The listing builds one solid part. Answer for the finished solid, in the listing's coordinates (mm). A direction names the side the tool comes from. Round coordinates to 2 decimals unless told otherwise and drop trailing zeros. Order: outer loops, then holes, each group sorted by start corner. A loop starts at its lowest first (then second) coordinate and runs counter-clockwise, first axis right, second up. Notation, with made-up numbers: (25, -9) - (62, -9) arc R27 ccw to (62, 13) - close; hole circle Ø7 at (64, 69). An arc over 180 degrees is marked (long way). Write item = value, one per line.
from build123d import *

# Parameters (mm, degrees)
SKETCH1_R           = 8
SKETCH1_R_2         = 3
BOSS_EXTRUDE1_DEPTH = 16.3
CHAMFER1_SIZE       = 0.1


with BuildPart() as part:
    # Sketch1 → Boss-Extrude1 (new, symmetric)
    with BuildSketch(Plane(origin=(0, 0, 0), x_dir=(0, 0, -1), z_dir=(1, 0, 0))):
        Circle(SKETCH1_R)
        Circle(SKETCH1_R_2, mode=Mode.SUBTRACT)
        Circle(SKETCH1_R_2)
    extrude(amount=BOSS_EXTRUDE1_DEPTH, both=True)

    # Sketch3 → M6 Tapped Hole1 (revolve, cut)
    with BuildSketch(Plane(origin=(-16.3, 0, 0), x_dir=(0, 0, 1), z_dir=(0, 1, 0))):
        Polygon((0, 0), (0, 11.502151548), (2.5, 10), (2.5, 0), align=None)
    m6_tapped_hole1 = revolve(axis=Axis((-22.65, 0, 0), (1, 0, 0)), mode=Mode.SUBTRACT)

    # Mirror1: M6 Tapped Hole1 across plane
    add(m6_tapped_hole1.mirror(Plane(origin=(0, 0, 0), x_dir=(0, 0, 1), z_dir=(1, 0, 0))), mode=Mode.SUBTRACT)

    # Chamfer1
    chamfer1_edges = [part.edges().sort_by_distance(p)[0] for p in [
        (-16.3, 0, 8),
        (16.3, 0, 8),
    ]]
    chamfer(chamfer1_edges, length=CHAMFER1_SIZE)


solid = part.part
Q1. For faces 4 (the face through (11.37, 2.44, -0.54)), 5 (the face through (-11.37, 2.44, -0.54)), 6 (the face through (-16.3, 2, 2)), determine the directions among +Z, -Z, +X, -X, +Y, -Y from which every point of the face is accessible in a straight line to the end or side of a thin tool.
Model answer:
face_4 = +X
face_5 = -X
face_6 = +Z, -Z, -X, +Y, -Y
Q2. Find the intervals of material crossed by line 1 (Y direction, x = 9, z = 0); line 2 (Z direction, x = -6.5, y = -1); line 3 (Z direction, x = 13.5, y = -0.25), in increasing order. Write a range as from..to.
Model answer:
line_1 = -8..-2.5, 2.5..8
line_2 = -7.94..-2.29, 2.29..7.94
line_3 = -8..-2.49, 2.49..8
Q3. Section A-A on x = 8 is taken. Determine the outline of the cut face in (y, z).
Model answer:
outline = circle Ø16 at (0, 0); hole circle Ø5 at (0, 0)
Q4. Section B-B on x = -3 is taken. Determine the outline of the cut face in (y, z), then the cut area to 3 significant figures.
Model answer:
outline = circle Ø16 at (0, 0)
area = 201 mm^2
Q5. Determine the mould class of faces 1 (the face through (5.059, 0.424, -0.094)), 2 (the face through (0.23, -7.81, 1.73)), 3 (the face through (16.3, 2, 2)) for opening direction Y: released by +Y, released by -Y, zero draft, split by the parting line, or undercut.
Model answer:
face_1 = undercut
face_2 = split by the parting line
face_3 = zero draft
Q6. A flat-ended cylindrical pin translates along its axis: P1, Ø1.5, axis at x = -9.5, z = -3, coming from the +Y side. Find the tip coordinate at first contact, or state that the pin passes through.
Model answer:
P1 = 7.68
